from build123d import *

# Parameters (mm, degrees)
SKETCH_1_W                  = 30
SKETCH_1_H                  = 36.2
EXTRUDE_1_DEPTH             = 8
CUT_EXTRUDE_1_DEPTH         = 48.691089314
CHAMFER_1_SIZE              = 2
CHAMFER_1_SIZE2             = 3.464101615
HOLE_WIZARD_M31_D           = 2.5
HOLE_WIZARD_M31_DEPTH       = 10.5
HOLE_WIZARD_M31_CSINK_D     = 3.3
HOLE_WIZARD_M31_CSINK_ANGLE = 110
HOLE_WIZARD_M31_TIP         = 0.751075774
HOLE_WIZARD_M32_D           = 2.5
HOLE_WIZARD_M32_DEPTH       = 10
HOLE_WIZARD_M32_CSINK_D     = 3.3
HOLE_WIZARD_M32_CSINK_ANGLE = 110
HOLE_WIZARD_M32_TIP         = 0.751075774


# Read off the part's stored shape, not the designer's step: Отверстие обработанное метчиком M35
with BuildPart() as part:
    # Эскиз1 → Бобышка-Вытянуть1 (new body)
    with BuildSketch(Plane.XY):
        with Locations((15, 18.1)):
            Rectangle(SKETCH_1_W, SKETCH_1_H)
    extrude(amount=EXTRUDE_1_DEPTH)

    # Эскиз2 → Вырез-Вытянуть1 (cut, through all)
    with BuildSketch(Plane(origin=(0, 0, 0), x_dir=(-1, 0, 0), z_dir=(0, 0, -1))):
        with BuildLine():
            Line((50.920424152, 122.962914197), (0, 34.766152423))
            Line((0, 34.766152423), (-11.660254038, 14.57))
            ThreePointArc((-11.660254038, 14.57), (-12.907797949, 8.215179054), (-10, 2.428571571))
            Line((-10, 2.428571571), (-10, 0))
            Line((-10, 0), (-10, -101.840848304))
            Line((-10, -101.840848304), (186.590983298, -155.115784424))
            Line((186.590983298, -155.115784424), (247.51140745, 69.687978076))
            Line((247.51140745, 69.687978076), (50.920424152, 122.962914197))
        make_face()
    extrude(amount=-CUT_EXTRUDE_1_DEPTH, mode=Mode.SUBTRACT)

    # Фаска1
    chamfer_1_edges = [part.edges().sort_by_distance(p)[0] for p in [
        (30, 18.1, 8),
    ]]
    chamfer_1_side = [part.faces().sort_by_distance(p)[0] for p in [
        (30, 18.1, 4),
    ]]
    chamfer(chamfer_1_edges, length=CHAMFER_1_SIZE, length2=CHAMFER_1_SIZE2, reference=chamfer_1_side[0])

    # Отверстие обработанное метчиком M31
    with Locations(Plane.XZ):
        with Locations((24, 5), (15, 5)):
            CounterSinkHole(HOLE_WIZARD_M31_D / 2, HOLE_WIZARD_M31_CSINK_D / 2, depth=HOLE_WIZARD_M31_DEPTH, counter_sink_angle=HOLE_WIZARD_M31_CSINK_ANGLE)
            with Locations((0, 0, -(HOLE_WIZARD_M31_DEPTH + HOLE_WIZARD_M31_TIP / 2))):  # 118° drill point
                Cone(0, HOLE_WIZARD_M31_D / 2, HOLE_WIZARD_M31_TIP, mode=Mode.SUBTRACT)

    # Отверстие обработанное метчиком M32
    with Locations(Plane(origin=(0, 36.2, 0), x_dir=(-1, 0, 0), z_dir=(0, 1, 0))):
        with Locations((-14, 5), (-26, 3)):
            CounterSinkHole(HOLE_WIZARD_M32_D / 2, HOLE_WIZARD_M32_CSINK_D / 2, depth=HOLE_WIZARD_M32_DEPTH, counter_sink_angle=HOLE_WIZARD_M32_CSINK_ANGLE)
            with Locations((0, 0, -(HOLE_WIZARD_M32_DEPTH + HOLE_WIZARD_M32_TIP / 2))):  # 118° drill point
                Cone(0, HOLE_WIZARD_M32_D / 2, HOLE_WIZARD_M32_TIP, mode=Mode.SUBTRACT)

    # Отверстие обработанное метчиком M35 outline → Отверстие обработанное метчиком M35 (revolve, cut)
    with BuildSketch(Plane(origin=(15, 23.2, 0), x_dir=(1, 0, 0), z_dir=(0, -1, 0))):
        Polygon((1.6, 8), (0, 8), (0, 0), (1.6, 0), (1.25, 0.245072638), (1.25, 7.754927362), align=None)
    revolve(axis=Axis((15, 23.2, 0), (0, 0, 1)), mode=Mode.SUBTRACT)

    # Hole Wizard M35 2 outline → Hole Wizard M35 2 (revolve, cut)
    with BuildSketch(Plane(origin=(27, 23.2, 0), x_dir=(1, 0, 0), z_dir=(0, -1, 0))):
        Polygon((1.6, 8), (0, 8), (0, 0), (1.6, 0), (1.25, 0.245072638), (1.25, 7.486978169), (1.6, 7.732050808), align=None)
    revolve(axis=Axis((27, 23.2, 0), (0, 0, 1)), mode=Mode.SUBTRACT)

    # Hole Wizard M35 3 outline → Hole Wizard M35 3 (revolve, cut)
    with BuildSketch(Plane(origin=(21, 17.2, 0), x_dir=(1, 0, 0), z_dir=(0, -1, 0))):
        Polygon((1.6, 8), (0, 8), (0, 0), (1.6, 0), (1.25, 0.245072638), (1.25, 7.754927362), align=None)
    revolve(axis=Axis((21, 17.2, 0), (0, 0, 1)), mode=Mode.SUBTRACT)

    # Hole Wizard M35 4 outline → Hole Wizard M35 4 (revolve, cut)
    with BuildSketch(Plane(origin=(21, 29.2, 0), x_dir=(1, 0, 0), z_dir=(0, -1, 0))):
        Polygon((1.6, 8), (0, 8), (0, 0), (1.6, 0), (1.25, 0.245072638), (1.25, 7.754927362), align=None)
    revolve(axis=Axis((21, 29.2, 0), (0, 0, 1)), mode=Mode.SUBTRACT)


solid = part.part
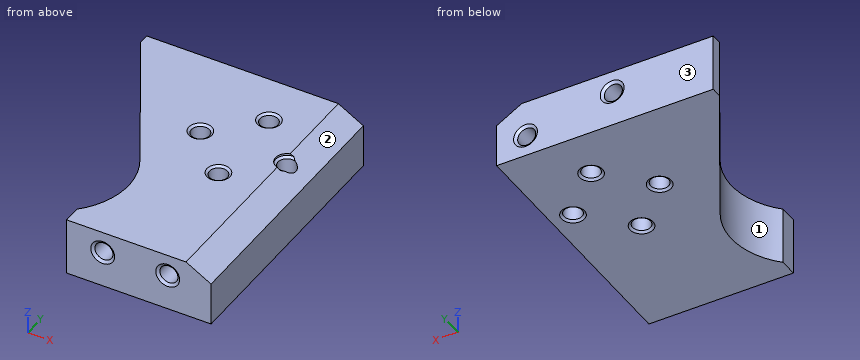
Check sheet for the modelled part. Datum: model origin and axes. Units: mm. Face numbers are marked on the shaded views. Round coordinates to 2 decimals unless told otherwise and drop trailing zeros. Order: outer loops, then holes, each group sorted by start corner. A loop starts at its lowest first (then second) coordinate and runs counter-clockwise, first axis right, second up.
Q1. Cross-section at D-D, the plane y = 23.2. Enter the section's corners in (x, z).
Filled sheet:
outline: (6.68, 0) - (13.4, 0) - (13.75, 0.25) - (13.75, 7.75) - (13.4, 8) - (6.68, 8) - close; (16.25, 0.25) - (16.6, 0) - (25.4, 0) - (25.75, 0.25) - (25.75, 7.49) - (25.4, 7.73) - (25.4, 8) - (16.6, 8) - (16.25, 7.75) - close; (28.25, 0.25) - (28.6, 0) - (30, 0) - (30, 6) - (28.25, 7.01) - close
Q2. Draft check along Y on the marked faces 1, 2 and 3. Enter one of: pulls with the +Y half, pulls with the -Y half, needs draft (parallel to the pull), parting line crosses it, or undercut.
Filled sheet:
face 1: undercut
face 2: needs draft
face 3: pulls with the +Y half
Q3. Cross-section at A-A, the plane x = 21. Enter the section's corners in (y, z), plus the area to 3 significant figures.
Filled sheet:
outline: (0, 0) - (15.6, 0) - (15.95, 0.25) - (15.95, 7.75) - (15.6, 8) - (0, 8) - close; (18.45, 0.25) - (18.8, 0) - (27.6, 0) - (27.95, 0.25) - (27.95, 7.75) - (27.6, 8) - (18.8, 8) - (18.45, 7.75) - close; (30.45, 0.25) - (30.8, 0) - (36.2, 0) - (36.2, 8) - (30.8, 8) - (30.45, 7.75) - close
area: 249 mm2
Q4. Depth check by flat-ended pin: P1, Ø3, axis at x = 26, z = 3, coming from the +Y side; P2, Ø1.2, axis at y = 1, z = 5, coming from the -X side; P3, Ø1, axis at y = 8.5, z = 6.5, coming from the -X side. Enter the tip coordinate at first touch or a pass-through.
Filled sheet:
P1: stops at y = 36.09
P2: stops at x = 10
P3: stops at x = 12.88
Q5. Cross-section at B-B, the plane y = 17.2. Enter the section's corners in (x, z).
Filled sheet:
outline: (10.14, 0) - (19.4, 0) - (19.75, 0.25) - (19.75, 7.75) - (19.4, 8) - (10.14, 8) - close; (22.25, 0.25) - (22.6, 0) - (30, 0) - (30, 6) - (26.54, 8) - (22.6, 8) - (22.25, 7.75) - close
Q6. Cross-section at C-C, the plane x = 11. Enter the section's corners in (y, z).
Filled sheet:
outline: (0, 0) - (3.57, 0) - (3.57, 8) - (0, 8) - close; (15.71, 0) - (36.2, 0) - (36.2, 8) - (15.71, 8) - close
Q7. Scan lines: L1, parallel to Y at x = 27, z = 6; L2, parallel to Y at x = 21, z = 3.5; L3, parallel to X at y = 23, z = 2.75. Record each from-to range of solid material in increasing order.
Filled sheet:
L1: y = 0 to 21.95, 24.45 to 36.2
L2: y = 0 to 15.95, 18.45 to 27.95, 30.45 to 36.2
L3: x = 6.79 to 13.77, 16.23 to 25.77, 28.23 to 30
